```python
from build123d import *

# Parameters (mm, degrees)
BOSS_EXTRUDE3_DEPTH = 4.42
BOSS_EXTRUDE4_DEPTH = 4.42
SKETCH7_W           = 4.13
SKETCH7_H           = 4.13
BOSS_EXTRUDE5_DEPTH = 0.7
SKETCH7_3_R         = 25.72
SKETCH7_3_R_2       = 16.51
SKETCH7_3_R_3       = 9.715
CUT_EXTRUDE1_DEPTH  = 1.2
SKETCH7_4_R         = 9.715
CUT_EXTRUDE2_DEPTH  = 2.76
FILLET2_R           = 2
SKETCH8_R           = 1.5
CUT_EXTRUDE3_DEPTH  = 106.505366688
SKETCH9_R           = 1.5
CUT_EXTRUDE4_DEPTH  = 106.473714261
SKETCH10_R          = 1.5
CUT_EXTRUDE5_DEPTH  = 106.473714261
SKETCH11_R          = 11
CUT_EXTRUDE6_DEPTH  = 106.473714261
FILLET7_R           = 10
SKETCH12_W          = 8.26
SKETCH12_H          = 8.26
CUT_EXTRUDE7_DEPTH  = 0.7


with BuildPart() as part:
    # Sketch6 → Boss-Extrude3 (new body)
    with BuildSketch(Plane(origin=(0, 0, 0), x_dir=(1, 0, 0), z_dir=(0, 1, 0))):
        Polygon((0, 0), (35.09, 0), (56.68, 0), (56.68, -56.68), (35.09, -56.68), (0, -56.68), align=None)
    extrude(amount=BOSS_EXTRUDE3_DEPTH)

    # Sketch6<7> → Boss-Extrude4 (add)
    with BuildSketch(Plane(origin=(0, 0, 0), x_dir=(1, 0, 0), z_dir=(0, 1, 0))):
        Polygon((35.09, 0), (56.68, 0), (88.84, 0), (88.84, 30), (35.09, 30), align=None)
    extrude(amount=BOSS_EXTRUDE4_DEPTH)

    # Sketch7 → Boss-Extrude5 (add)
    with BuildSketch(Plane(origin=(0, 4.42, 0), x_dir=(1, 0, 0), z_dir=(0, 1, 0))):
        with Locations((26.275, -30.405)):
            Rectangle(SKETCH7_W, SKETCH7_H)
        with Locations((26.275, -26.275)):
            Rectangle(SKETCH7_W, SKETCH7_H)
        with Locations((30.405, -26.275)):
            Rectangle(SKETCH7_W, SKETCH7_H)
        with Locations((30.405, -30.405)):
            Rectangle(SKETCH7_W, SKETCH7_H)
    extrude(amount=BOSS_EXTRUDE5_DEPTH)

    # Sketch7<3> → Cut-Extrude1 (cut)
    # profile 1 of 2: a face of its own
    with BuildSketch(Plane(origin=(0, 4.42, 0), x_dir=(1, 0, 0), z_dir=(0, 1, 0))):
        with Locations(Location((28.34, -28.34, 0), (0, 0, 270))):
            Circle(SKETCH7_3_R)
        with Locations((28.34, -28.34)):
            Circle(SKETCH7_3_R_2, mode=Mode.SUBTRACT)
    # profile 2 of 2: a face of its own
    with BuildSketch(Plane(origin=(0, 4.42, 0), x_dir=(1, 0, 0), z_dir=(0, 1, 0))):
        with Locations((28.34, -28.34)):
            Circle(SKETCH7_3_R_2)
        with Locations(Location((28.34, -28.34, 0), (0, 0, 270))):
            Circle(SKETCH7_3_R_3, mode=Mode.SUBTRACT)
    extrude(amount=-CUT_EXTRUDE1_DEPTH, mode=Mode.SUBTRACT)

    # Sketch7<4> → Cut-Extrude2 (cut)
    with BuildSketch(Plane(origin=(0, 4.42, 0), x_dir=(1, 0, 0), z_dir=(0, 1, 0))):
        with Locations(Location((28.34, -28.34, 0), (0, 0, 270))):
            Circle(SKETCH7_4_R)
        Polygon((24.21, -28.34), (24.21, -32.47), (28.34, -32.47), (32.47, -32.47), (32.47, -28.34), (32.47, -24.21), (28.34, -24.21), (24.21, -24.21), align=None, mode=Mode.SUBTRACT)
    extrude(amount=-CUT_EXTRUDE2_DEPTH, mode=Mode.SUBTRACT)

    # Fillet2
    fillet2_edges = [part.edges().sort_by_distance(p)[0] for p in [
        (32.47, 3.39, 32.47),
        (32.47, 3.39, 24.21),
        (24.21, 3.39, 24.21),
        (24.21, 3.39, 32.47),
    ]]
    fillet(fillet2_edges, radius=FILLET2_R)

    # Sketch8 → Cut-Extrude3 (cut, through all)
    with BuildSketch(Plane(origin=(0, 5.12, 0), x_dir=(1, 0, 0), z_dir=(0, 1, 0))):
        with Locations(Location((28.34, -28.34, 0), (0, 0, 270))):
            Circle(SKETCH8_R)
    extrude(amount=-CUT_EXTRUDE3_DEPTH, mode=Mode.SUBTRACT)

    # Sketch9 → Cut-Extrude4 (cut, through all)
    with BuildSketch(Plane(origin=(0, 4.42, 0), x_dir=(1, 0, 0), z_dir=(0, 1, 0))):
        with Locations(Location((5, -5, 0), (0, 0, 270))):
            Circle(SKETCH9_R)
        with Locations(Location((51.68, -5, 0), (0, 0, 270))):
            Circle(SKETCH9_R)
        with Locations(Location((51.68, -51.68, 0), (0, 0, 270))):
            Circle(SKETCH9_R)
        with Locations(Location((5, -51.68, 0), (0, 0, 270))):
            Circle(SKETCH9_R)
    extrude(amount=-CUT_EXTRUDE4_DEPTH, mode=Mode.SUBTRACT)

    # Sketch10 → Cut-Extrude5 (cut, through all)
    with BuildSketch(Plane(origin=(0, 4.42, 0), x_dir=(1, 0, 0), z_dir=(0, 1, 0))):
        with Locations(Location((40.09, 25, 0), (0, 0, 270))):
            Circle(SKETCH10_R)
        with Locations(Location((40.09, 5, 0), (0, 0, 270))):
            Circle(SKETCH10_R)
        with Locations(Location((83.84, 5, 0), (0, 0, 270))):
            Circle(SKETCH10_R)
        with Locations(Location((83.84, 25, 0), (0, 0, 270))):
            Circle(SKETCH10_R)
        with BuildLine():
            Line((45.69, 26.5), (48.69, 26.5))
            ThreePointArc((48.69, 26.5), (50.19, 25), (48.69, 23.5))
            Line((48.69, 23.5), (45.69, 23.5))
            ThreePointArc((45.69, 23.5), (44.19, 25), (45.69, 26.5))
        make_face()
        with BuildLine():
            Line((45.69, 6.5), (48.69, 6.5))
            ThreePointArc((48.69, 6.5), (50.19, 5), (48.69, 3.5))
            Line((48.69, 3.5), (45.69, 3.5))
            ThreePointArc((45.69, 3.5), (44.19, 5), (45.69, 6.5))
        make_face()
    extrude(amount=-CUT_EXTRUDE5_DEPTH, mode=Mode.SUBTRACT)

    # Sketch11 → Cut-Extrude6 (cut, through all)
    with BuildSketch(Plane(origin=(0, 4.42, 0), x_dir=(1, 0, 0), z_dir=(0, 1, 0))):
        with Locations(Location((68.84, 15.364869593, 0), (0, 0, 270))):
            Circle(SKETCH11_R)
    extrude(amount=-CUT_EXTRUDE6_DEPTH, mode=Mode.SUBTRACT)

    # Fillet7
    fillet7_edges = [part.edges().sort_by_distance(p)[0] for p in [
        (35.09, 2.21, 0),
        (56.68, 2.21, 0),
    ]]
    fillet(fillet7_edges, radius=FILLET7_R)

    # Sketch12 → Cut-Extrude7 (cut)
    with BuildSketch(Plane(origin=(0, 5.12, 0), x_dir=(1, 0, 0), z_dir=(0, 1, 0))):
        with Locations((28.34, -28.34)):
            Rectangle(SKETCH12_W, SKETCH12_H)
    extrude(amount=-CUT_EXTRUDE7_DEPTH, mode=Mode.SUBTRACT)


solid = part.part
```
Geometry check sheet. Reference: the model listing, model coordinates, mm. A direction names the side the tool comes from. Round coordinates to 2 decimals unless told otherwise and drop trailing zeros. Loops run counter-clockwise (first coordinate to the right, second up) from the corner with the lowest first, then second, coordinate; pieces in that order, holes last. Notation, with made-up numbers: (4.25, 24) - (9.25, 24) arc R14 ccw to (9.25, 50) - close; hole circle Ø4 at (55.25, 20). An arc over 180 degrees is marked (long way). Use a Markdown table: item, result.
Q1. Cross-section at C-C on x = 68.84. Record the cut outline in (y, z).
Solutions:
| item | result |
|---|---|
| outline | (0, -30) - (4.42, -30) - (4.42, -26.36) - (0, -26.36) - close; (0, -4.36) - (4.42, -4.36) - (4.42, 0) - (0, 0) - close |
Q2. Draft check along X on faces 4 (the cylindrical face through (50.19, 2.24, -25.03)), 5 (the cylindrical face through (44.19, 2.24, -24.97)), 6 (the flat face through (0, 2, 29)), 7 (the flat face through (78, 2, 0)). Enter one of: released by +X, released by -X, zero draft, split by the parting line, or undercut.
Solutions:
| item | result |
|---|---|
| face 4 | undercut |
| face 5 | undercut |
| face 6 | released by -X |
| face 7 | zero draft |
Q3. Material ranges on line 1 (X direction, y = 3.1, z = -25); line 2 (X direction, y = 2.8, z = 4); line 3 (Z direction, x = 52, y = 1.85), recorded low to high.
Solutions:
| item | result |
|---|---|
| line 1 | x = 35.09 to 38.59, 41.59 to 44.19, 50.19 to 63.53, 74.15 to 82.34, 85.34 to 88.84 |
| line 2 | x = 0 to 3.88, 6.12 to 50.56, 52.8 to 58.68 |
| line 3 | z = -30 to 3.53, 6.47 to 50.21, 53.15 to 56.68 |
Q4. Access from +Z, -Z, +X, -X, +Y, -Y to the whole of each face (thin tool, end or side, straight path). Record for faces 1 (the flat face through (32.47, 3, 28)), 2 (the flat face through (47, 2, -26.5)), 3 (the flat face through (34, 0, 13)).
Solutions:
| item | result |
|---|---|
| face 1 | +Y |
| face 2 | +Y, -Y |
| face 3 | +Z, -Z, +X, -X, -Y |
Q5. Cross-section at D-D on y = 0.9. State how many separate pieces and enclosed holes the cut face has, plus the area to 3 significant figures.
Solutions:
| item | result |
|---|---|
| separate pieces | 1 |
| enclosed holes | 12 |
| area | 4,390 mm2 |
Q6. Cross-section at B-B on z = 28.34. Record the cut outline in (x, y) (3 decimals).
Solutions:
| item | result |
|---|---|
| outline | (0, 0) - (26.84, 0) - (26.84, 4.42) - (24.21, 4.42) - (24.21, 1.66) - (18.625, 1.66) - (18.625, 3.22) - (2.62, 3.22) - (2.62, 4.42) - (0, 4.42) - close; (29.84, 0) - (56.68, 0) - (56.68, 4.42) - (54.06, 4.42) - (54.06, 3.22) - (38.055, 3.22) - (38.055, 1.66) - (32.47, 1.66) - (32.47, 4.42) - (29.84, 4.42) - close |
Q7. Go/stop test with flat-tipped pins: P1, Ø2, axis at x = 48, z = 19, coming from the +Y side; P2, Ø12, axis at x = 29, z = 35.5, coming from the +Y side; P3, Ø2, axis at x = 17, y = 1, coming from the -Z side; P4, Ø2, axis at y = 1.5, z = -24.5, coming from the -X side. Record where each tip stops, or that it passes through.
Solutions:
| item | result |
|---|---|
| P1 | stops at y = 3.22 |
| P2 | stops at y = 4.42 |
| P3 | stops at z = 0 |
| P4 | stops at x = 35.09 |
Q8. Cross-section at A-A on x = 83.84. Record the cut outline in (y, z), plus the area to 3 significant figures.
Solutions:
| item | result |
|---|---|
| outline | (0, -30) - (4.42, -30) - (4.42, -26.5) - (0, -26.5) - close; (0, -23.5) - (4.42, -23.5) - (4.42, -6.5) - (0, -6.5) - close; (0, -3.5) - (4.42, -3.5) - (4.42, 0) - (0, 0) - close |
| area | 106 mm2 |
